Geometry: see drawing. Coordinates: mm, zero at the bounding-box minimum. Round coordinates to 2 decimals unless told otherwise and drop trailing zeros. Loops run counter-clockwise (first coordinate to the right, second up) from the corner with the lowest first, then second, coordinate; pieces in that order, holes last. Notation, with made-up numbers: (-14.75, -7) - (41.25, -7) arc R30 ccw to (41.25, 27) - close; hole circle Ø9 at (-39.5, 82.25). An arc over 180 degrees is marked (long way). One line per question, with ' | ' between items. Start each with the question number.
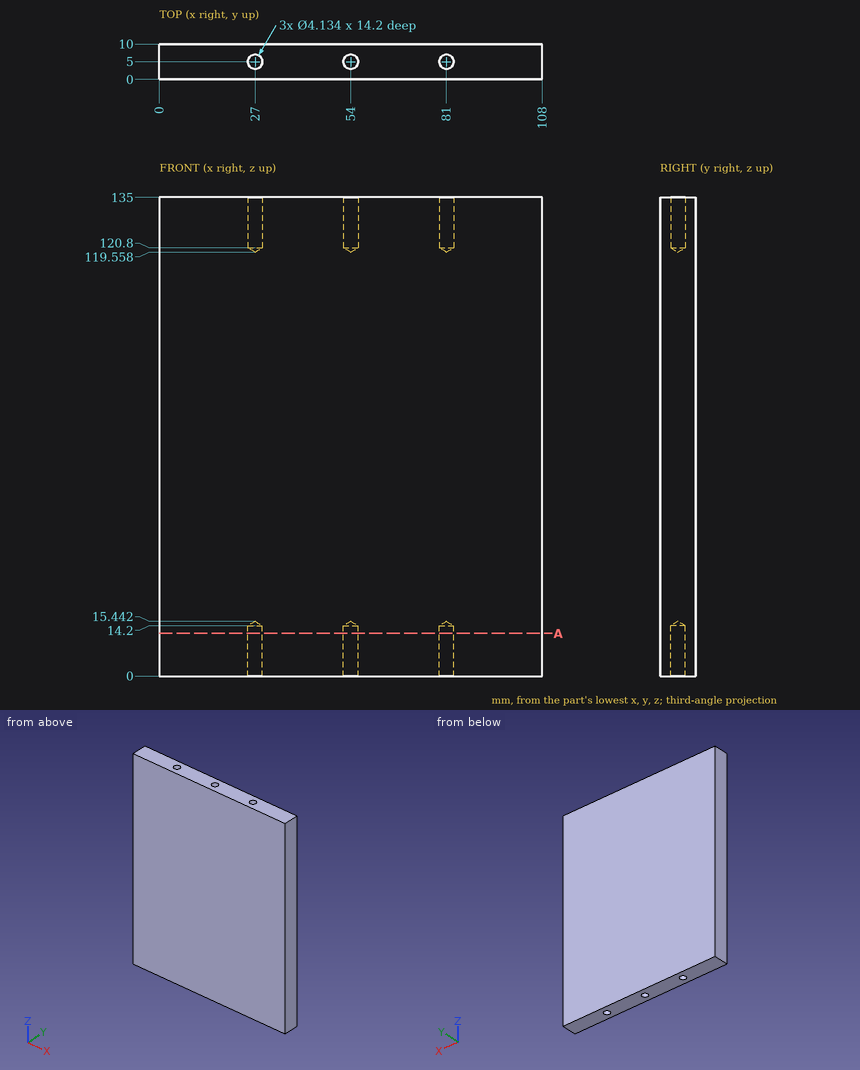
(1) Line query: line 1 along X through (y, z) = (5, 9.5); line 2 along Y through (x, z) = (54, 128.25); line 3 along Z through (x, y) = (25.5, 6). Output: solid intervals per line, ascending. Write a range as from..to.
(2) Section A-A, the plane z = 12. Output: boundary loops of the cut face in (x, y).
(3) Pin query (flat end, axial travel): P1, Ø3.5, axis at x = 81, y = 5, coming from the -Z side; P2, Ø2.5, axis at x = 54, y = 5, coming from the +Z side. Return the tip coordinate at first contact, or that it passes through.
Derived:
1) line 1: x = 0..24.93, 29.07..51.93, 56.07..78.93, 83.07..108 | line 2: y = 0..2.93, 7.07..10 | line 3: z = 14.36..120.64
2) outline: (0, 0) - (108, 0) - (108, 10) - (0, 10) - close; hole circle Ø4.13 at (27, 5); hole circle Ø4.13 at (54, 5); hole circle Ø4.13 at (81, 5)
3) P1: stops at z = 14.39 | P2: stops at z = 120.31
